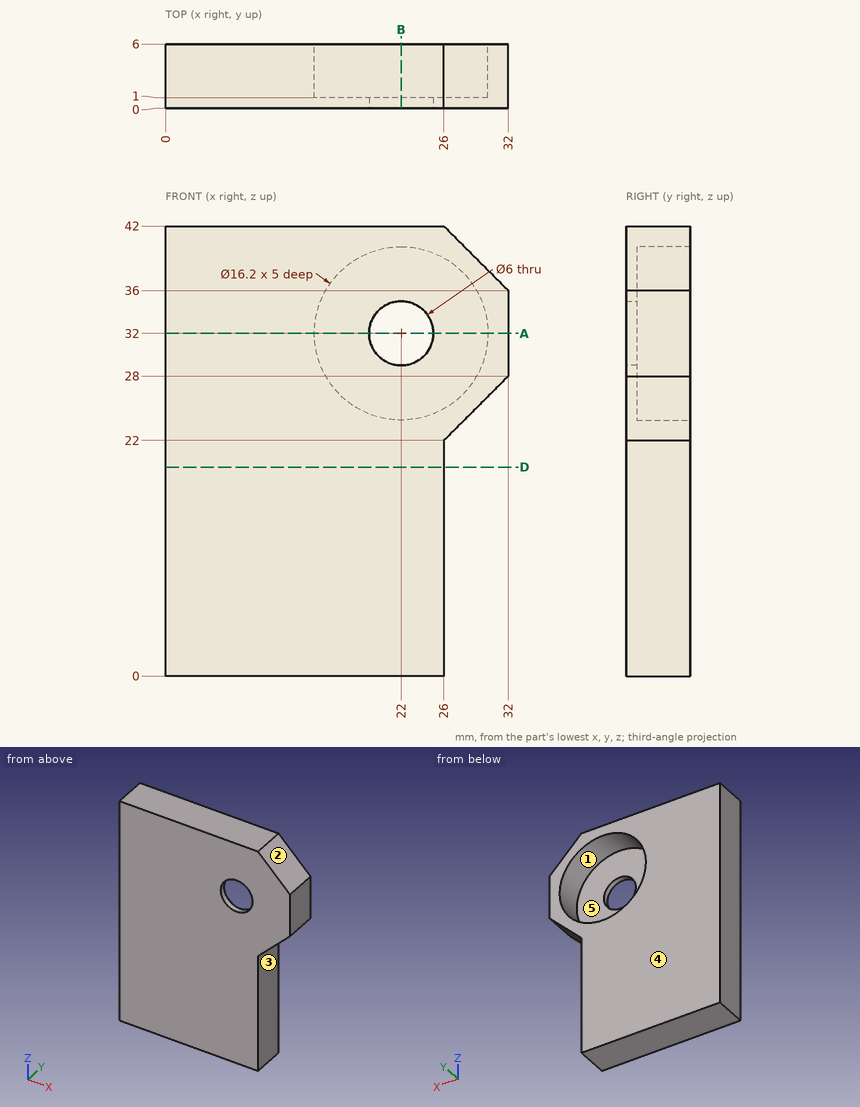
Here's the drawing with two shaded views (mm, measured from the low corner). I have some questions. A direction names the side the tool comes from. Coordinates: 2 decimals unless noted, no trailing zeros. Loops run counter-clockwise (first coordinate to the right, second up) from the corner with the lowest first, then second, coordinate; pieces in that order, holes last. Notation, with made-up numbers: M 7,-27 L 60,-27 A11 cw 60,-9 Z; hole C 72,7 d1. An arc over 180 degrees is marked long. Return JSON: item names as keys, results as strings. Group by question number.
Item 1: Imagine slicing it at A-A (z = 32). Please give me the cut outline in (x, y).
Item 2: If I drill on L1, parallel to Z at x = 22, y = 0.3; L2, parallel to X at y = 0.2, z = 32; L3, parallel to X at y = 2.35, z = 32, over which ranges is the centre line in solid material (lowest first)? Write a range as from..to.
Item 3: Thinking about a two-plate mould opening in Z: for the marked faces 1, 2 and 3, which applies, released by +Z, released by -Z, zero draft, split by the parting line, or undercut?
Item 4: Imagine slicing it at B-B (x = 22). Please give me the cut outline in (y, z).
Item 5: On a 3-axis mill with a long thin cutter (end or side, diameter ignored), from which of +Z, -Z, +X, -X, +Y, -Y can I reach the whole of each face in a straight line? I mean the marked faces 4 and 5. Say none if no direction works.
Item 6: Imagine slicing it at D-D (z = 19.5). Please give me the cut outline in (x, y), and give its area (3 significant figures).
Item 7: I'm going to push a flat-ended pin straight in: pin 1 Ø9.5 at (x, z) = (22, 32) entering from +Y. Where does the tip first touch, or does it pass through?
Verdict:
{
 "1": {"outline": "M 0,0 L 19,0 L 19,1 L 13.9,1 L 13.9,6 L 0,6 Z; M 25,0 L 32,0 L 32,6 L 30.1,6 L 30.1,1 L 25,1 Z"},
 "2": {"L1": "z = 0..29, 35..42", "L2": "x = 0..19, 25..32", "L3": "x = 0..13.9, 30.1..32"},
 "3": {"face 1": "undercut", "face 2": "released by +Z", "face 3": "zero draft"},
 "4": {"outline": "M 0,0 L 6,0 L 6,23.9 L 1,23.9 L 1,29 L 0,29 Z; M 0,35 L 1,35 L 1,40.1 L 6,40.1 L 6,42 L 0,42 Z"},
 "5": {"face 4": "+Z, -Z, +X, -X, +Y", "face 5": "+Y"},
 "6": {"outline": "M 0,0 L 26,0 L 26,6 L 0,6 Z", "area": "156 mm^2"},
 "7": {"pin 1": "stops at y = 1"}
}
